```python
from build123d import *

# Parameters (mm, degrees)
F1_DEPTH = 50.8
F3_D     = 50.8
F4_R     = 3.175


# Not quite as in the source:
# - a feature of the source that left no trace in its solid (it failed there, or was rolled back) is left out


with BuildPart() as f1:
    # F0 (on Right) → F1 (new body)
    with BuildSketch(Plane.YZ):
        Polygon((208.5787526399, 38.1), (-70.8212473601, 38.1), (5.3787526399, -38.1), (132.3787526399, -38.1), align=None)
    extrude(amount=F1_DEPTH)

    # F3 (through all)
    with Locations(Plane(origin=(0, 0, 0), x_dir=(0, 1, 0), z_dir=(-1, 0, 0))):
        with Locations((68.8787526399, 0)):
            Hole(F3_D / 2)

    # F4
    f4_edges = [f1.edges().sort_by_distance(p)[0] for p in [
        (0, 68.878753, 38.1),
        (25.4, 5.378753, -38.1),
        (0, 68.878753, -38.1),
        (50.8, 68.878753, -38.1),
        (25.4, -70.821247, 38.1),
        (0, -32.721247, 0),
        (50.8, -32.721247, 0),
        (25.4, 208.578753, 38.1),
        (0, 170.478753, 0),
        (50.8, 170.478753, 0),
        (50.8, 68.878753, 38.1),
    ]]
    fillet(f4_edges, radius=F4_R)


solid = f1.part
```
Read the model definition and answer for the solid it produces. Units are mm, in the model's axes. Coordinates: 2 decimals unless noted, no trailing zeros. Loops run counter-clockwise (first coordinate to the right, second up) from the corner with the lowest first, then second, coordinate; pieces in that order, holes last.
(1) The part is cut by section B-B (y = 61). Determine the outline of the cut face in (x, z) (3 decimals).
Solution:
outline: (0, -34.925) arc R3.175 ccw to (3.175, -38.1) - (47.625, -38.1) arc R3.175 ccw to (50.8, -34.925) - (50.8, -24.147) - (0, -24.147) - close; (0, 24.147) - (50.8, 24.147) - (50.8, 34.925) arc R3.175 ccw to (47.625, 38.1) - (3.175, 38.1) arc R3.175 ccw to (0, 34.925) - close
(2) Consider line 1 along Z through (x, y) = (21, 50.5); line 2 along Z through (x, y) = (5, 80); line 3 along Y through (x, z) = (41, 18.5). Determine where each line is inside the solid, lowest interval first.
Solution:
line 1: z = -38.1 to -17.53, 17.53 to 38.1
line 2: z = -38.1 to -22.84, 22.84 to 38.1
line 3: y = -51.22 to 51.47, 86.28 to 188.98
(3) The part is cut by section A-A (x = 37). Determine the outline of the cut face in (y, z) (3 decimals), and give its area (3 significant figures).
Solution:
outline: (-65.401, 32.68) - (4.449, -37.17) arc R3.175 ccw to (6.694, -38.1) - (132.379, -38.1) - (203.159, 32.68) arc R3.175 ccw to (200.914, 38.1) - (-63.156, 38.1) arc R3.175 ccw to start; hole circle Ø50.8 at (68.879, 0)
area: 13,400 mm2
(4) The mould has two halves that part along Z. Classify faces 1 (the face through (0, 67, 32)), 2 (the face through (0.95, 167.62, -1.57)), 3 (the face through (25.8, 89, 15.5)): released by +Z, released by -Z, zero draft, split by the parting line, or undercut.
Solution:
face 1: zero draft
face 2: released by -Z
face 3: undercut
(5) Flat-ended cylindrical pins translate along their axes: pin 1 Ø2 at (x, y) = (28.5, 152.5) entering from -Z; pin 2 Ø4 at (x, z) = (33, 21) entering from -Y; pin 3 Ø6 at (x, z) = (35, -12) entering from -Y. Find the tip coordinate at first contact, or state that the pin passes through.
Solution:
pin 1: stops at z = -18.98
pin 2: stops at y = -55.72
pin 3: stops at y = -23.72
